```python
from build123d import *

# Parameters (mm, degrees)
BOSS_EXTRU_1_DEPTH      = 350
ESQUISSE2_W             = 100
ESQUISSE2_H             = 100
BOSS_EXTRU_2_DEPTH      = 430
ENL_V_MAT_EXTRU_1_DEPTH = 570.758720863
ESQUISSE4_R             = 2.5
ENL_V_MAT_EXTRU_2_DEPTH = 570.758720863


with BuildPart() as part:
    # Esquisse1 → Boss.-Extru.1 (new body)
    with BuildSketch(Plane(origin=(0, 0, 0), x_dir=(1, 0, 0), z_dir=(0, 1, 0))):
        Polygon((-165, 60), (0, 175.570498661), (165, 60), (165, -60), (91.241437954, -150), (-91.241437954, -150), (-165, -60), align=None)
    extrude(amount=BOSS_EXTRU_1_DEPTH)

    # Esquisse2 → Boss.-Extru.2 (add)
    with BuildSketch(Plane(origin=(0, 0, 0), x_dir=(1, 0, 0), z_dir=(0, 1, 0))):
        Rectangle(ESQUISSE2_W, ESQUISSE2_H)
    extrude(amount=BOSS_EXTRU_2_DEPTH)

    # Esquisse3 → Enlèv. mat.-Extru.1 (cut, through all)
    with BuildSketch(Plane(origin=(165, 0, 0), x_dir=(0, 0, -1), z_dir=(1, 0, 0))):
        Polygon((175.570498661, 0), (120, 0), (120, 280), (65, 280), (65, 340), (175.570498661, 340), align=None)
    extrude(amount=-ENL_V_MAT_EXTRU_1_DEPTH, mode=Mode.SUBTRACT)

    # Esquisse4 → Enlèv. mat.-Extru.2 (cut, through all)
    with BuildSketch(Plane(origin=(165, 0, 0), x_dir=(0, 0, -1), z_dir=(1, 0, 0))):
        with Locations((-40, 330)):
            Circle(ESQUISSE4_R)
    extrude(amount=-ENL_V_MAT_EXTRU_2_DEPTH, mode=Mode.SUBTRACT)


solid = part.part
```
Part model, mm, in its own coordinate system. A direction names the side the tool comes from. Round coordinates to 2 decimals unless told otherwise and drop trailing zeros. Write each loop counter-clockwise with the first axis right and the second up, starting at its lowest first coordinate (ties: lowest second). Pieces come first, ordered by that corner, then holes. Notation, with made-up numbers: (74.25, 64.5) -> (88.25, 64.5) arc R23 ccw to (88.25, 77.5) -> close; hole circle Ø10 at (43.5, 45). An arc over 180 degrees is marked (long way). Return JSON: item names as keys, results as strings. Group by question number.
Q1. Probe L1, parallel to Y at x = 20, z = 40; L2, parallel to Z at x = 74, y = 330; L3, parallel to Y at x = 61, z = 40. List the from-to ranges inside material, lowest first. Write a range as [from, to].
Q2. Saw through at B-B on z = -81.5. Write the cut outline in (x, y).
Q3. Saw through at A-A on y = 219.5. Write the cut outline in (x, z), plus the area to 3 significant figures.
Q4. Saw through at D-D on z = 3.5. Write the cut outline in (x, y).
Q5. Saw through at C-C on x = -127.5. Write the cut outline in (y, z), plus the area to 3 significant figures.
Q6. Pin check, flat tips, straight feed: pin 1 (24 mm diameter, centred on x = 7, y = 392.5, fed in from -Z); pin 2 (6 mm diameter, centred on x = 113.5, y = 49, fed in from -Z); pin 3 (3 mm diameter, centred on x = -49.5, y = 147.5, fed in from -Z); pin 4 (5 mm diameter, centred on x = -27, z = 60.5, fed in from -Y). Stop position of each tip, or through.
Q7. Which spindle directions (+Z, -Z, +X, -X, +Y, -Y) get a long thin tool onto all of the face, cutting with end or side? Do faces 1 (the flat face through (-1, 389, -50)), 2 (the flat face through (-1, 389, 50)), 3 (the flat face through (2, 340, -107)). Say none if no direction does.
Answer:
{
 "1": {"L1": "[0, 327.5], [332.5, 430]", "L2": "[-65, 37.5], [42.5, 150]", "L3": "[0, 327.5], [332.5, 350]"},
 "2": {"outline": "(-134.3, 0) -> (134.3, 0) -> (134.3, 280) -> (-134.3, 280) -> close; (-134.3, 340) -> (134.3, 340) -> (134.3, 350) -> (-134.3, 350) -> close"},
 "3": {"outline": "(-165, -60) -> (-79.34, -120) -> (79.34, -120) -> (165, -60) -> (165, 60) -> (91.24, 150) -> (-91.24, 150) -> (-165, 60) -> close", "area": "77,300 mm2"},
 "4": {"outline": "(-165, 0) -> (165, 0) -> (165, 350) -> (50, 350) -> (50, 430) -> (-50, 430) -> (-50, 350) -> (-165, 350) -> close"},
 "5": {"outline": "(0, -86.27) -> (280, -86.27) -> (280, -65) -> (340, -65) -> (340, -86.27) -> (350, -86.27) -> (350, 105.76) -> (0, 105.76) -> close; hole circle Ø5 at (330, 40)", "area": "65,900 mm2"},
 "6": {"pin 1": "z = -50", "pin 2": "z = -98.17", "pin 3": "z = -120", "pin 4": "y = 0"},
 "7": {"face 1": "-Z, +X, -X, +Y", "face 2": "+Z, +X, -X, +Y", "face 3": "-Z, +X, -X"}
}
